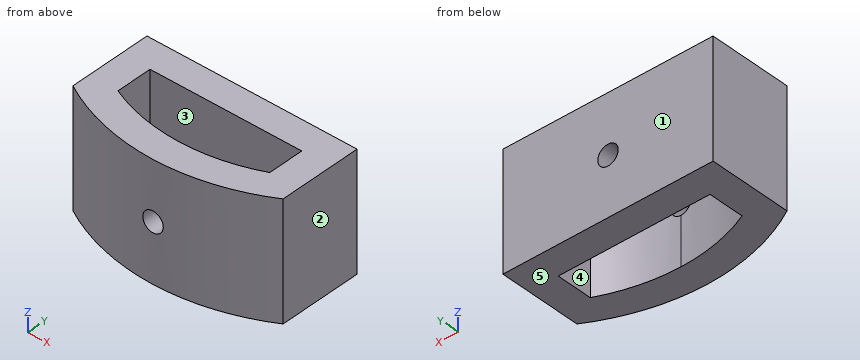
```python
from build123d import *

# Parameters (mm, degrees)
BOSS_EXTRUDE1_DEPTH = 10
SKETCH2_R           = 0.875
CUT_EXTRUDE3_DEPTH  = 23


with BuildPart() as part:
    # Sketch1 → Boss-Extrude1 (new body)
    with BuildSketch(Plane.XY):
        with BuildLine():
            ThreePointArc((6.5, -14.071247279), (3.327586751, -15.138598562), (0, -15.5))
            ThreePointArc((0, -15.5), (-3.327586751, -15.138598562), (-6.5, -14.071247279))
            ThreePointArc((-6.5, -14.071247279), (-7.783922131, -13.403751574), (-9, -12.619429464))
            Line((-9, -12.619429464), (-9, -15.588457268))
            ThreePointArc((-9, -15.588457268), (0, -18), (9, -15.588457268))
            Line((9, -15.588457268), (9, -12.619429464))
            ThreePointArc((9, -12.619429464), (7.783922131, -13.403751574), (6.5, -14.071247279))
        make_face()
        with BuildLine():
            Line((-6.5, -11), (0, -11))
            Line((0, -11), (0, -8.5))
            Line((0, -8.5), (-9, -8.5))
            Line((-9, -8.5), (-9, -12.619429464))
            ThreePointArc((-9, -12.619429464), (-7.783922131, -13.403751574), (-6.5, -14.071247279))
            Line((-6.5, -14.071247279), (-6.5, -12.619429464))
            Line((-6.5, -12.619429464), (-6.5, -11))
        make_face()
        with BuildLine():
            Line((0, -8.5), (0, -11))
            Line((0, -11), (6.5, -11))
            Line((6.5, -11), (6.5, -12.619429464))
            Line((6.5, -12.619429464), (6.5, -14.071247279))
            ThreePointArc((6.5, -14.071247279), (7.783922131, -13.403751574), (9, -12.619429464))
            Line((9, -12.619429464), (9, -8.5))
            Line((9, -8.5), (0, -8.5))
        make_face()
    extrude(amount=BOSS_EXTRUDE1_DEPTH)

    # Sketch2 → Cut-Extrude3 (cut)
    with BuildSketch(Plane(origin=(0, 0, 0), x_dir=(1, 0, 0), z_dir=(0, 1, 0))):
        with Locations((0, -5)):
            Circle(SKETCH2_R)
    extrude(amount=-CUT_EXTRUDE3_DEPTH, mode=Mode.SUBTRACT)


solid = part.part
```
Geometry: final body of the model. Coordinates: model frame, mm. Face numbers are marked on the shaded views. A direction names the side the tool comes from. Coordinates: 2 decimals unless noted, no trailing zeros. Order: outer loops, then holes, each group sorted by start corner. A loop starts at its lowest first (then second) coordinate and runs counter-clockwise, first axis right, second up. Notation, with made-up numbers: (21.5, -25.75) -> (42.5, -25.75) arc R25 cw to (42.5, 4.25) -> close; hole circle Ø8 at (30, 70.5). An arc over 180 degrees is marked (long way). Answer in a Markdown table with one row per item.
Item 1: Draft query along X for the marked faces 1, 2 and 3. Return one class per face: released by +X, released by -X, zero draft, split by the parting line, or undercut.
Return value:
| item | result |
|---|---|
| face 1 | zero draft |
| face 2 | released by +X |
| face 3 | undercut |
Item 2: Access query for the marked faces 4 and 5. Directions: +Z, -Z, +X, -X, +Y, -Y. A direction counts if a zero-diameter tool reaches every point of the face in a straight line with its end or side. Return the directions, or none.
Return value:
| item | result |
|---|---|
| face 4 | +Z, -Z |
| face 5 | -Z, +X, -X, +Y, -Y |
Item 3: Ray query, L1, parallel to X at y = -12.5, z = 7.25; L2, parallel to Z at x = 0, y = -9.8 (3 decimals); L3, parallel to X at y = -9.5, z = 5 (3 decimals). Return the intervals inside material, ascending.
Return value:
| item | result |
|---|---|
| L1 | x = -9 to -6.5, 6.5 to 9 |
| L2 | z = 0 to 4.125, 5.875 to 10 |
| L3 | x = -9 to -0.875, 0.875 to 9 |
Item 4: Section B-B on x = 0.5. Output: boundary loops of the cut face in (y, z), plus the area to 3 significant figures.
Return value:
| item | result |
|---|---|
| outline | (-17.99, 0) -> (-15.49, 0) -> (-15.49, 4.28) -> (-17.99, 4.28) -> close; (-17.99, 5.72) -> (-15.49, 5.72) -> (-15.49, 10) -> (-17.99, 10) -> close; (-11, 0) -> (-8.5, 0) -> (-8.5, 4.28) -> (-11, 4.28) -> close; (-11, 5.72) -> (-8.5, 5.72) -> (-8.5, 10) -> (-11, 10) -> close |
| area | 42.8 mm² |
Item 5: Section C-C on y = -15. Output: boundary loops of the cut face in (x, z), plus the area to 3 significant figures.
Return value:
| item | result |
|---|---|
| outline | (-9, 0) -> (-3.91, 0) -> (-3.91, 10) -> (-9, 10) -> close; (3.91, 0) -> (9, 0) -> (9, 10) -> (3.91, 10) -> close |
| area | 102 mm² |
Item 6: Section A-A on z = 1.75. Output: boundary loops of the cut face in (x, y).
Return value:
| item | result |
|---|---|
| outline | (-9, -15.59) arc R18 ccw to (9, -15.59) -> (9, -8.5) -> (-9, -8.5) -> close; hole (-6.5, -14.07) arc R15.5 ccw to (6.5, -14.07) -> (6.5, -11) -> (-6.5, -11) -> close |
Item 7: Section D-D on z = 4.75. Output: boundary loops of the cut face in (x, y), plus the area to 3 significant figures.
Return value:
| item | result |
|---|---|
| outline | (-9, -15.59) arc R18 ccw to (-0.84, -17.98) -> (-0.84, -15.48) arc R15.5 cw to (-6.5, -14.07) -> (-6.5, -11) -> (-0.84, -11) -> (-0.84, -8.5) -> (-9, -8.5) -> close; (0.84, -17.98) arc R18 ccw to (9, -15.59) -> (9, -8.5) -> (0.84, -8.5) -> (0.84, -11) -> (6.5, -11) -> (6.5, -14.07) arc R15.5 cw to (0.84, -15.48) -> close |
| area | 96.1 mm² |
Item 8: Contact query for a flat-ended pin moving along its axis: P1, Ø1, axis at y = -16.5, z = 8.5, coming from the -X side. Output: stop coordinate, or through.
Return value:
| item | result |
|---|---|
| P1 | stops at x = -8.25 |
